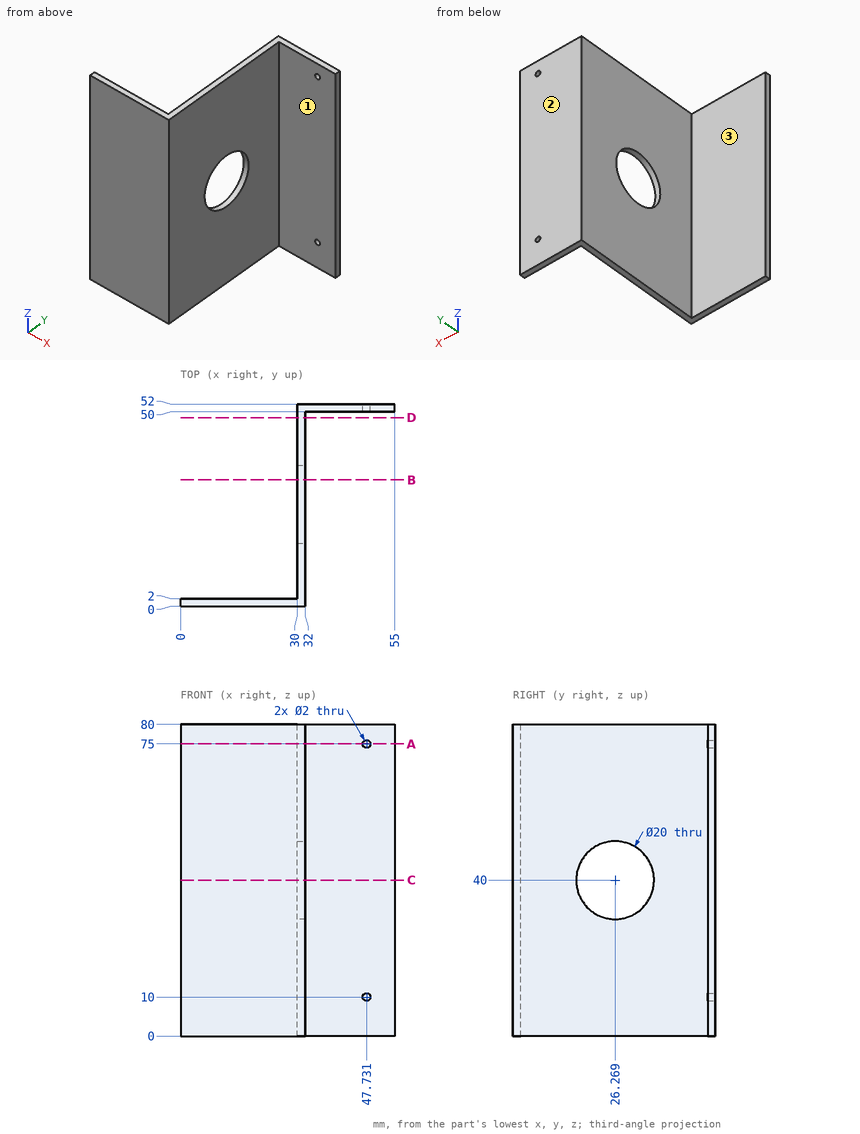
The figure shows three views and two pictorial views of one solid part (mm, origin at its lowest corner). Answer the questions. A direction names the side the tool comes from. Round coordinates to 2 decimals unless told otherwise and drop trailing zeros. Write each loop counter-clockwise with the first axis right and the second up, starting at its lowest first coordinate (ties: lowest second). Pieces come first, ordered by that corner, then holes. Notation, with made-up numbers: (73.25, 89) - (127.25, 89) arc R7 cw to (127.25, 93) - close; hole circle Ø9 at (49, -32.75). An arc over 180 degrees is marked (long way). Answer in a Markdown table with one row per item. Add a question column.
1. Given pin 1 (1.5 mm diameter, centred on y = 42, z = 32.5, fed in from +X); pin 2 (7 mm diameter, centred on x = 41.5, z = 39, fed in from -Y); pin 3 (2.5 mm diameter, centred on x = 47.73, z = 75, fed in from +Y); pin 4 (3 mm diameter, centred on y = 46.5, z = 62, fed in from -X), each flat-ended and moving along its own axis, determine where each tip first touches the part or whether it passes through.
2. Find the intervals of material crossed by line 1 along X through (y, z) = (51.4, 10); line 2 along Y through (x, z) = (30.45, 40); line 3 along X through (y, z) = (22.5, 50.5), in increasing order. Write a range as from..to.
3. A cutting plane is placed at D-D, the plane y = 48.5. Determine the outline of the cut face in (x, z), and give its area (3 significant figures).
4. For the marked faces 1, 2 and 3, determine the directions among +Z, -Z, +X, -X, +Y, -Y from which every point of the face is accessible in a straight line to the end or side of a thin tool.
5. A cutting plane is placed at A-A, the plane z = 75. Determine the outline of the cut face in (x, y).
6. A cutting plane is placed at C-C, the plane z = 40. Determine the outline of the cut face in (x, y).
7. A cutting plane is placed at B-B, the plane y = 32.5. Determine the outline of the cut face in (x, z).
Worked out:
| question | item | result |
|---|---|---|
| 1 | pin 1 | x = 32 |
| 1 | pin 2 | y = 50 |
| 1 | pin 3 | y = 52 |
| 1 | pin 4 | x = 30 |
| 2 | line 1 | 30..46.73, 48.73..55 |
| 2 | line 2 | 0..16.27, 36.27..52 |
| 2 | line 3 | 30..32 |
| 3 | outline | (30, 0) - (32, 0) - (32, 80) - (30, 80) - close |
| 3 | area | 160 mm^2 |
| 4 | face 1 | +Z, -Z, +X, -Y |
| 4 | face 2 | +Z, -Z, +X, -X, +Y |
| 4 | face 3 | +Z, -Z, -X, +Y |
| 5 | outline | (0, 0) - (32, 0) - (32, 50) - (46.73, 50) - (46.73, 52) - (30, 52) - (30, 2) - (0, 2) - close; (48.73, 50) - (55, 50) - (55, 52) - (48.73, 52) - close |
| 6 | outline | (0, 0) - (32, 0) - (32, 16.27) - (30, 16.27) - (30, 2) - (0, 2) - close; (30, 36.27) - (32, 36.27) - (32, 50) - (55, 50) - (55, 52) - (30, 52) - close |
| 7 | outline | (30, 0) - (32, 0) - (32, 32.18) - (30, 32.18) - close; (30, 47.82) - (32, 47.82) - (32, 80) - (30, 80) - close |
